Source: CAD feature listing. Evaluate the final solid. Frame: model axes, mm. Face numbers are marked on the shaded views. A direction names the side the tool comes from. Give positions to 0.01 mm unless a question says otherwise; leave off trailing zeros. Loops run counter-clockwise (first coordinate to the right, second up) from the corner with the lowest first, then second, coordinate; pieces in that order, holes last. Notation, with made-up numbers: M 29.25,55 L 85.25,55 A20 ccw 85.25,65 Z; hole C -33,60 d1. An arc over 180 degrees is marked long. Write item = value, one per line.
from build123d import *

# Parameters (mm, degrees)
F0_W      = 101.6
F0_H      = 101.6
F1_DEPTH  = 35.56
F2_R      = 13.75
F2_R_2    = 11.43
F5_DEPTH  = 66.04
F6_DEPTH  = 81.28
F4_R      = 10.3
F4_R_2    = 10.570977
F4_R_3    = 6.35
F7_DEPTH  = 25.4
F3_R      = 6.35
F8_DEPTH  = 50.8
F3_R_2    = 10.3
F3_R_3    = 10.675077
F9_DEPTH  = 25.4
F10_DEPTH = 38.1


with BuildPart() as f1:
    # F0 (on Top) → F1 (new body)
    with BuildSketch(Plane.XY):
        with Locations((50.8, 50.8)):
            Rectangle(F0_W, F0_H)
    extrude(amount=F1_DEPTH)

    # F2 (on face) → F5 (cut)
    with BuildSketch(Plane.XZ):
        with Locations((63.5, 17.78)):
            Circle(F2_R)
        with Locations((63.5, 17.78)):
            Circle(F2_R_2, mode=Mode.SUBTRACT)
        with Locations((63.5, 17.78)):
            Circle(F2_R_2)
    extrude(amount=-F5_DEPTH, mode=Mode.SUBTRACT)

    # F2 (on face) → F6 (cut)
    with BuildSketch(Plane.XZ):
        with Locations((63.5, 17.78)):
            Circle(F2_R_2)
    extrude(amount=-F6_DEPTH, mode=Mode.SUBTRACT)

    # F4 (on face) → F7 (cut)
    with BuildSketch(Plane.YZ.offset(101.6)):
        with Locations((21.59, 17.78)):
            Circle(F4_R)
        with Locations((78.74, 17.78)):
            Circle(F4_R_2)
        with Locations((78.74, 17.78)):
            Circle(F4_R_3, mode=Mode.SUBTRACT)
    extrude(amount=-F7_DEPTH, mode=Mode.SUBTRACT)

    # F3 (on face) → F8 (cut)
    with BuildSketch(Plane(origin=(0, 0, 0), x_dir=(0, -1, 0), z_dir=(-1, 0, 0))):
        with Locations((-60.96, 17.78)):
            Circle(F3_R)
        with Locations((-22.86, 17.78)):
            Circle(F3_R)
    extrude(amount=-F8_DEPTH, mode=Mode.SUBTRACT)

    # F3 (on face) → F9 (cut)
    with BuildSketch(Plane(origin=(0, 0, 0), x_dir=(0, -1, 0), z_dir=(-1, 0, 0))):
        with Locations((-60.96, 17.78)):
            Circle(F3_R_2)
        with Locations((-60.96, 17.78)):
            Circle(F3_R, mode=Mode.SUBTRACT)
        with Locations((-22.86, 17.78)):
            Circle(F3_R_3)
        with Locations((-22.86, 17.78)):
            Circle(F3_R, mode=Mode.SUBTRACT)
    extrude(amount=-F9_DEPTH, mode=Mode.SUBTRACT)

    # F4 (on face) → F10 (cut)
    with BuildSketch(Plane.YZ.offset(101.6)):
        with Locations((78.74, 17.78)):
            Circle(F4_R_3)
    extrude(amount=-F10_DEPTH, mode=Mode.SUBTRACT)


solid = f1.part
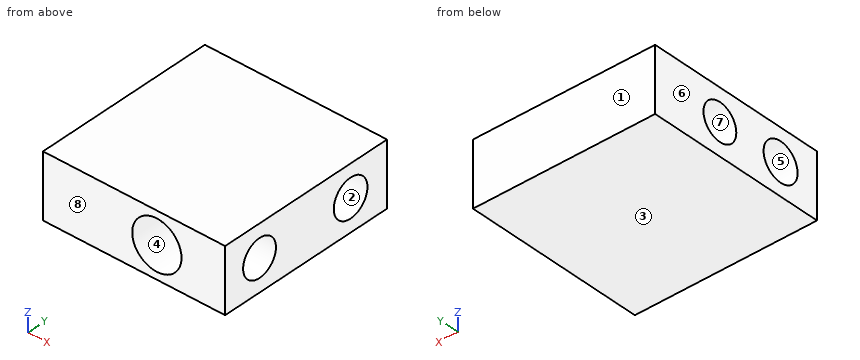
1. Cut plane A-A, the plane y = 60.96. Return the cut outline in (x, z), then the cut area to 3 significant figures.
Derived:
outline = M 0,0 L 101.6,0 L 101.6,35.56 L 0,35.56 L 0,28.08 L 25.4,28.08 L 25.4,24.13 L 50.8,24.13 L 50.8,23.05 A13.75 cw long 50.8,12.51 L 50.8,11.43 L 25.4,11.43 L 25.4,7.48 L 0,7.48 Z
area = 2,180 mm²
2. Cut plane C-C, the plane x = 92. Return the cut outline in (y, z), then the cut area to 3 significant figures.
Derived:
outline = M 0,0 L 101.6,0 L 101.6,35.56 L 0,35.56 Z; hole C 21.59,17.78 d20.6; hole C 78.74,17.78 d21.14
area = 2,930 mm²
3. Pull-direction query (Y, two-part tool) for the marked faces 6, 7 and 8; classes: +Y half, -Y half, draft (parallel to the pull), parting line (faces both ways), or undercut.
Derived:
face_6 = draft
face_7 = undercut
face_8 = -Y half
4. First-contact query: pin 1 Ø10 at (y, z) = (77, 22) entering from +X; pin 2 Ø12 at (x, z) = (65.5, 22.5) entering from -Y; pin 3 Ø2 at (y, z) = (82.5, 19.5) entering from +X. Flat tips, straight axial feed; report the tip coordinate or a pass-through.
Derived:
pin_1 = 76.2
pin_2 = 81.28
pin_3 = 63.5
5. Cut plane D-D, the plane z = 17.78. Count the separate pieces of the cut face and the enclosed holes in it, then the cut area to 3 significant figures.
Derived:
separate_pieces = 5
enclosed_holes = 0
area = 5,370 mm²
6. Reachability of the marked faces 1, 2, 3, 4 and 5 from +Z, -Z, +X, -X, +Y, -Y: full face, straight path, thin tool, end or side. Return the list, or none.
Derived:
face_1 = +Z, -Z, +X, -X, +Y
face_2 = +X
face_3 = -Z, +X, -X, +Y, -Y
face_4 = -Y
face_5 = -X
7. Material intervals for probe 1 along Y at (x, z) = (90, 17); probe 2 along Z at (x, y) = (63.5, 39); probe 3 along Y at (x, z) = (77, 23.5), sorted ascending. Write a range as from..to.
Derived:
probe_1 = 0..11.32, 31.86..68.2, 89.28..101.6
probe_2 = 0..4.03, 31.53..35.56
probe_3 = 0..13.02, 30.16..69.85, 87.63..101.6
8. Cut plane B-B, the plane y = 21.59. Return the cut outline in (x, z), then the cut area to 3 significant figures.
Derived:
outline = M 0,0 L 101.6,0 L 101.6,7.48 L 76.2,7.48 L 76.2,12.51 A13.75 cw 50.8,12.51 L 50.8,11.56 L 25.4,11.56 L 25.4,7.18 L 0,7.18 Z; M 0,28.38 L 25.4,28.38 L 25.4,24 L 50.8,24 L 50.8,23.05 A13.75 cw 76.2,23.05 L 76.2,28.08 L 101.6,28.08 L 101.6,35.56 L 0,35.56 Z
area = 1,660 mm²
